from build123d import *

# Parameters (mm, degrees)
F2_R = 1


with BuildPart() as f1:
    # F0 (on Front) → F1 (revolve)
    with BuildSketch(Plane.XZ):
        Polygon((-19.4, 0), (-5, 0), (-5, 1.4), (-11.25, 1.4), (-11.25, 7.4), (-12.8, 7.4), (-12.8, 1.4), (-16.4, 1.4), (-16.4, 3.4), (-19.4, 2.001077), align=None)
    revolve(axis=Axis((0, 0, 4.390553), (0, 0, 1)))

    # F2
    f2_edges = [f1.edges().sort_by_distance(p)[0] for p in [
        (19.4, 0, 2.001077),
        (19.4, 0, 0),
    ]]
    fillet(f2_edges, radius=F2_R)


solid = f1.part
Geometry: final body of the model. Coordinates: model frame, mm. A direction names the side the tool comes from. Give positions to 0.01 mm unless a question says otherwise; leave off trailing zeros. Loops run counter-clockwise (first coordinate to the right, second up) from the corner with the lowest first, then second, coordinate; pieces in that order, holes last. Notation, with made-up numbers: (-34, 82) - (-11, 82) arc R19 ccw to (-11, 87) - close; hole circle Ø6 at (82.5, 50.5). An arc over 180 degrees is marked (long way). Answer as CSV lines item,"result". Start each with the question number.
1. Section A-A, the plane z = 5. Return loops of the section in (x, y).
2. Pin query (flat end, axial travel): P1, Ø3, axis at y = -6, z = 2.5, coming from the +X side; P2, Ø2, axis at y = 10, z = 6, coming from the +X side; P3, Ø10, axis at x = -11.5, y = -11.5, coming from the +Z side; P4, Ø4, axis at x = 0.5, z = 5, coming from the -Y side. Return the tip coordinate at first contact, or that it passes through.
3. Ray query, L1, parallel to X at y = 0, z = 2.4; L2, parallel to X at y = 0, z = 3.15; L3, parallel to Y at x = -0.5, z = 1.75. Return the intervals inside material, ascending.
4. Draft query along X for faces 3 (the face through (-9, 10, 1.4)), 4 (the face through (-17.92, 7.43, 1.18)), 5 (the face through (-4, 4, 0)). Return one class per face: released by +X, released by -X, zero draft, split by the parting line, or undercut.
5. Reachability of faces 1 (the face through (2, 5, 1.4)), 2 (the face through (4.7, 10.4, 7.4)) from +Z, -Z, +X, -X, +Y, -Y: full face, straight path, thin tool, end or side. Return the list, or none.
Answers:
1,outline,"circle Ø25.6 at (0, 0); hole circle Ø22.5 at (0, 0)"
2,P1,"stops at x = 18.77"
2,P2,"stops at x = 9.1"
2,P3,"stops at z = 7.4"
2,P4,"stops at y = -17.25"
3,L1,"x = -18.54 to -16.4, -12.8 to -11.25, 11.25 to 12.8, 16.4 to 18.54"
3,L2,"x = -16.94 to -16.4, -12.8 to -11.25, 11.25 to 12.8, 16.4 to 16.94"
3,L3,"y = -19.32 to -16.39, -12.79 to -11.24, 11.24 to 12.79, 16.39 to 19.32"
4,face 3,"undercut"
4,face 4,"split by the parting line"
4,face 5,"zero draft"
5,face 1,"+Z"
5,face 2,"+Z, +X, -X, +Y, -Y"
